Here's how the part is built. I have some questions about the finished solid (model axes, mm). A direction names the side the tool comes from. Give positions to 0.01 mm unless a question says otherwise; leave off trailing zeros. Write each loop counter-clockwise with the first axis right and the second up, starting at its lowest first coordinate (ties: lowest second). Pieces come first, ordered by that corner, then holes. Notation, with made-up numbers: M -35,-23.75 L -9,-23.75 A34 ccw -9,15.25 Z; hole C 50,-33 d10. An arc over 180 degrees is marked long. Use one line per item in the form item = value. Start each with the question number.
from build123d import *

# Parameters (mm, degrees)
MAIN_DEPTH        = 3.2
WHEEL_DEPTH       = 3.2
SKETCH3_W         = 25
SKETCH3_H         = 5
TABS_DEPTH        = 3.2
SCREW_HOLES_DEPTH = 3.2
SKETCH6_W         = 16
SKETCH6_H         = 11
USB_HOLE_DEPTH    = 3.2


with BuildPart() as part:
    # Sketch1 → main (new body)
    with BuildSketch(Plane(origin=(0, 0, 0), x_dir=(0, 0, -1), z_dir=(1, 0, 0))):
        with BuildLine():
            Line((-87.535437106, 0), (122.464562894, 0))
            Line((122.464562894, 0), (122.464562894, 30))
            add(Edge.make_bspline(
                [(-87.535437106, 20), (17.331032425, 30.296907598), (122.464562894, 30)],
                knots=[0, 0, 0, 1, 1, 1], degree=2))
            Line((-87.535437106, 20), (-87.535437106, 0))
        make_face()
    extrude(amount=MAIN_DEPTH)

    # Sketch2 → wheel (cut)
    with BuildSketch(Plane(origin=(3.2, 0, 0), x_dir=(0, 0, -1), z_dir=(1, 0, 0))):
        with BuildLine():
            Line((-87.535437106, 0), (-54.535437106, 0))
            Line((-54.535437106, 0), (-54.535437106, 4))
            ThreePointArc((-54.535437106, 4), (-57.464369294, 11.071067812), (-64.535437106, 14))
            Line((-64.535437106, 14), (-87.535437106, 14))
            Line((-87.535437106, 14), (-87.535437106, 0))
        make_face()
    extrude(amount=-WHEEL_DEPTH, mode=Mode.SUBTRACT)

    # Sketch3 → tabs (add)
    with BuildSketch(Plane(origin=(3.2, 0, 0), x_dir=(0, 0, -1), z_dir=(1, 0, 0))):
        with Locations((-25.035437106, -2.5)):
            Rectangle(SKETCH3_W, SKETCH3_H)
        with Locations((99.964562894, -2.5)):
            Rectangle(SKETCH3_W, SKETCH3_H)
    extrude(amount=-TABS_DEPTH)

    # Sketch5 → screw holes (cut)
    with BuildSketch(Plane(origin=(3.2, 0, 0), x_dir=(0, 0, -1), z_dir=(1, 0, 0))):
        Polygon((7.464562894, 0), (10.264562894, 0), (10.264562894, 9.7), (11.664562894, 9.7), (11.664562894, 12), (10.264562894, 12), (10.264562894, 17), (7.464562894, 17), (7.464562894, 12), (6.064562894, 12), (6.064562894, 9.7), (7.464562894, 9.7), align=None)
        Polygon((60.264562894, 0), (63.064562894, 0), (63.064562894, 9.7), (64.464562894, 9.7), (64.464562894, 12), (63.064562894, 12), (63.064562894, 17), (60.264562894, 17), (60.264562894, 12), (58.864562894, 12), (58.864562894, 9.7), (60.264562894, 9.7), align=None)
    extrude(amount=-SCREW_HOLES_DEPTH, mode=Mode.SUBTRACT)

    # Sketch6 → USB hole (cut)
    with BuildSketch(Plane(origin=(3.2, 0, 0), x_dir=(0, 0, -1), z_dir=(1, 0, 0))):
        with Locations((-34.535437106, 9.5)):
            Rectangle(SKETCH6_W, SKETCH6_H)
    extrude(amount=-USB_HOLE_DEPTH, mode=Mode.SUBTRACT)


solid = part.part
1) Thinking about a two-plate mould opening in Y: for faces 1 (the face through (2, 14, -63.065)), 2 (the face through (2, 9, 26.535)), 3 (the face through (2, -5, -100)), which applies, released by +Y, released by -Y, zero draft, split by the parting line, or undercut?
2) Suppose I cut it at A-A, the plane y = 6. List the corners of the cut face in (x, z) for me, and give its area (3 significant figures).
3) Please list where these lines run through material, in increasing order: line 1 (Z direction, x = 2.55, y = 3); line 2 (Z direction, x = 1.95, y = 5); line 3 (Y direction, x = 2.9, z = 1.5).
4) On a 3-axis mill with a long thin cutter (end or side, diameter ignored), from which of +Z, -Z, +X, -X, +Y, -Y can I reach the whole of each face in a straight line? I mean faces 4 (the face through (2, 15, -122.465)), 5 (the face through (2, 14, 76)), 6 (the face through (2, 5, -7.465)), 7 (the face through (2, 9, 42.535)), 8 (the face through (2, 0, -117)). Say none if no direction works.
5) Will these pins go through, and if not, where does the flat tip stop? P1, Ø1, axis at x = 2, y = 3.5, coming from the +Z side; P2, Ø1.1, axis at x = 1, z = -63.5, coming from the -Y side; P3, Ø10, axis at y = 12, z = -77.5, coming from the -X side; P4, Ø1.5, axis at x = 2.5, z = -60, coming from the +Y side.
Checks:
q1.face_1 = zero draft
q1.face_2 = undercut
q1.face_3 = released by -Y
q2.outline = M 0,-122.46 L 3.2,-122.46 L 3.2,-63.06 L 0,-63.06 Z; M 0,-60.26 L 3.2,-60.26 L 3.2,-10.26 L 0,-10.26 Z; M 0,-7.46 L 3.2,-7.46 L 3.2,26.54 L 0,26.54 Z; M 0,42.54 L 3.2,42.54 L 3.2,54.74 L 0,54.74 Z
q2.area = 498 mm^2
q3.line_1 = -122.46 to -63.06, -60.26 to -10.26, -7.46 to 54.54
q3.line_2 = -122.46 to -63.06, -60.26 to -10.26, -7.46 to 26.54, 42.54 to 54.59
q3.line_3 = 0 to 26.66
q4.face_4 = -Z, +X, -X, +Y, -Y
q4.face_5 = +Z, +X, -X, -Y
q4.face_6 = +X, -X, -Y
q4.face_7 = +X, -X
q4.face_8 = -Z, +X, -X, -Y
q5.P1 = 54.54
q5.P2 = 0
q5.P3 = 0
q5.P4 = 29.26
